from build123d import *

# Parameters (mm, degrees)
SKETCH1_W                = 69.825
SKETCH1_H                = 183.16
FRONT_PLATE_DEPTH        = 1.2
CUT_EXTRUDE1_REACH       = 197.283
SKETCH3_W                = 56.825
SKETCH3_H                = 78.5
SKETCH3_H_2              = 48.66
CONVERT_SOLID5_START     = 1.1684
CONVERT_SOLID5_DEPTH     = 0.0316
M3_CLEARANCE_HOLE1_D     = 3.2
M3_CLEARANCE_HOLE1_DEPTH = 5
M3_CLEARANCE_HOLE1_TIP   = 0.96137699
SKETCH62_W               = 13
SKETCH62_H               = 78.5
BOSS_EXTRUDE2_DEPTH      = 1.1684
FILLET1_R                = 5
M3_CLEARANCE_HOLE2_D     = 3.2
M3_CLEARANCE_HOLE2_DEPTH = 5
M3_CLEARANCE_HOLE2_TIP   = 0.96137699


# Read off the part's stored shape, not the designer's step: Convert-Solid5
with BuildPart() as part:
    # Sketch1 → front_plate (new body)
    with BuildSketch(Plane.XY):
        with Locations((34.9125, -90.788691865)):
            Rectangle(SKETCH1_W, SKETCH1_H)
    extrude(amount=FRONT_PLATE_DEPTH)

    # Sketch3 → Cut-Extrude1 (cut, up to next)
    with BuildSketch(Plane.XY.offset(1.2), mode=Mode.PRIVATE) as cut_extrude1_sk1:
        with Locations((28.4125, -68.458691865)):
            Rectangle(SKETCH3_W, SKETCH3_H)
    cut_extrude1_tool1 = extrude(cut_extrude1_sk1.sketch, amount=-CUT_EXTRUDE1_REACH, mode=Mode.PRIVATE) & part.part
    # Sketch3 → Cut-Extrude1 (cut, up to next)
    with BuildSketch(Plane.XY.offset(1.2), mode=Mode.PRIVATE) as cut_extrude1_sk2:
        with Locations((28.4125, -145.038691865)):
            Rectangle(SKETCH3_W, SKETCH3_H_2)
    cut_extrude1_tool2 = extrude(cut_extrude1_sk2.sketch, amount=-CUT_EXTRUDE1_REACH, mode=Mode.PRIVATE) & part.part
    add(cut_extrude1_tool1.solids().sort_by_distance((28.4125, -68.458692, 1.2))[0], mode=Mode.SUBTRACT)
    add(cut_extrude1_tool2.solids().sort_by_distance((28.4125, -145.038692, 1.2))[0], mode=Mode.SUBTRACT)

    # Convert-Solid5 outline → Convert-Solid5 (cut)
    with BuildSketch(Plane.XY.offset(CONVERT_SOLID5_START)):
        Polygon((56.825, -107.708691865), (0, -107.708691865), (0, -120.708691865), (56.825, -120.708691865), (56.825, -169.368691865), (0, -169.368691865), (0, -182.368691865), (69.825, -182.368691865), (69.825, 0.791308135), (0, 0.791308135), (0, -29.208691865), (56.825, -29.208691865), align=None)
    extrude(amount=CONVERT_SOLID5_DEPTH, mode=Mode.SUBTRACT)

    # M3 Clearance Hole1
    with Locations(Plane.XY.offset(1.1684)):
        with Locations((63.325, -92.708691865), (63.325, -113.708691865), (64.2, -6.233691865), (64.2, -175.343691865)):
            Hole(M3_CLEARANCE_HOLE1_D / 2, depth=M3_CLEARANCE_HOLE1_DEPTH)
            with Locations((0, 0, -(M3_CLEARANCE_HOLE1_DEPTH + M3_CLEARANCE_HOLE1_TIP / 2))):  # 118° drill point
                Cone(0, M3_CLEARANCE_HOLE1_D / 2, M3_CLEARANCE_HOLE1_TIP, mode=Mode.SUBTRACT)

    # Mirror2: part across plane


with BuildPart() as part_1:
    add(part.part)
    add(part.part.mirror(Plane(origin=(0, 0.791308135, 0), x_dir=(0, 0, 1), z_dir=(-1, 0, 0))))

    # Sketch62 → Boss-Extrude2 (add)
    with BuildSketch(Plane.XY.offset(1.1684)):
        with Locations((-8.74, -68.458691865)):
            Rectangle(SKETCH62_W, SKETCH62_H)
    extrude(amount=-BOSS_EXTRUDE2_DEPTH)

    # Fillet1
    fillet1_edges = [part_1.edges().sort_by_distance(p)[0] for p in [
        (-15.24, -107.708691865, 0.5842),
        (-15.24, -29.208691865, 0.5842),
        (-2.24, -29.208691865, 0.5842),
        (-2.24, -107.708691865, 0.5842),
        (56.825, -120.708691865, 0.5842),
        (56.825, -169.368691865, 0.5842),
        (69.825, -182.368691865, 0.5842),
        (69.825, 0.791308135, 0.5842),
        (56.825, -29.208691865, 0.5842),
        (56.825, -107.708691865, 0.5842),
        (-56.825, -107.708691865, 0.5842),
        (-56.825, -29.208691865, 0.5842),
        (-69.825, 0.791308135, 0.5842),
        (-69.825, -182.368691865, 0.5842),
        (-56.825, -169.368691865, 0.5842),
        (-56.825, -120.708691865, 0.5842),
    ]]
    fillet(fillet1_edges, radius=FILLET1_R)

    # M3 Clearance Hole2
    with Locations(Plane.XY.offset(1.1684)):
        with Locations((-8.74, -6.233691865), (-8.74, -59.958691865), (-8.74, -113.708691865)):
            Hole(M3_CLEARANCE_HOLE2_D / 2, depth=M3_CLEARANCE_HOLE2_DEPTH)
            with Locations((0, 0, -(M3_CLEARANCE_HOLE2_DEPTH + M3_CLEARANCE_HOLE2_TIP / 2))):  # 118° drill point
                Cone(0, M3_CLEARANCE_HOLE2_D / 2, M3_CLEARANCE_HOLE2_TIP, mode=Mode.SUBTRACT)


solid = part_1.part
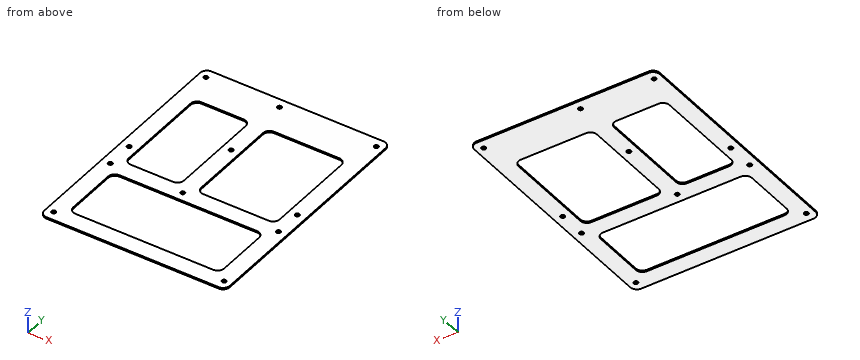
Design review of the part built by this model. Coordinates are the model's own, in mm. Give positions to 0.01 mm unless a question says otherwise; leave off trailing zeros. Loops run counter-clockwise (first coordinate to the right, second up) from the corner with the lowest first, then second, coordinate; pieces in that order, holes last. Notation, with made-up numbers: (12.25, 5.5) - (30.25, 5.5) arc R20 ccw to (30.25, 22.5) - close; hole circle Ø10 at (-5.75, -9.75). An arc over 180 degrees is marked (long way). Use CSV: the item, a comma, the result in double quotes. Start each with the question number.
1. Add section D-D (z = 0.2). Count the separate pieces of the cut face and the enclosed holes in it, plus the area to 3 significant figures.
2. Insertion check: P1, Ø3, axis at x = 63.32, y = -92.71, coming from the -Z side; P2, Ø4, axis at x = -63.32, y = -92.71, coming from the -Z side. Each pin has a flat end and moves straight along its axis. Give the tip position at first contact, or say it passes through.
3. Add section C-C (x = -29.5). State the section outline as (y, z) points, plus the area to 3 significant figures.
4. Wall thickness on L1, parallel to X at y = -65, z = 0.2 (3 decimals); L2, parallel to Y at x = -8.74, z = 0.5; L3, parallel to Y at x = 2.5, z = 0.55: over which ranges is each line inside the solid? List them lowest first.
5. Add section B-B (y = -149). State the section outline as (x, z) points (3 decimals), plus the area to 3 significant figures.
6. Add section A-A (y = -43.5). State the section outline as (x, z) points (3 decimals), plus the area to 3 significant figures.
Results found:
1,separate pieces,"1"
1,enclosed holes,"14"
1,area,"12,100 mm²"
2,P1,"passes through"
2,P2,"stops at z = 0"
3,outline,"(-182.37, 0) - (-169.37, 0) - (-169.37, 1.17) - (-182.37, 1.17) - close; (-120.71, 0) - (-107.71, 0) - (-107.71, 1.17) - (-120.71, 1.17) - close; (-29.21, 0) - (0.79, 0) - (0.79, 1.17) - (-29.21, 1.17) - close"
3,area,"65.4 mm²"
4,L1,"x = -69.825 to -56.825, -15.24 to -2.24, 56.825 to 69.825"
4,L2,"y = -182.37 to -169.37, -120.71 to -115.31, -112.11 to -61.56, -58.36 to -7.83, -4.63 to 0.79"
4,L3,"y = -182.37 to -169.37, -120.71 to -107.7, -29.22 to 0.79"
5,outline,"(-69.825, 0) - (-56.825, 0) - (-56.825, 1.168) - (-69.825, 1.168) - close; (56.825, 0) - (69.825, 0) - (69.825, 1.168) - (56.825, 1.168) - close"
5,area,"30.4 mm²"
6,outline,"(-69.825, 0) - (-56.825, 0) - (-56.825, 1.168) - (-69.825, 1.168) - close; (-15.24, 0) - (-2.24, 0) - (-2.24, 1.168) - (-15.24, 1.168) - close; (56.825, 0) - (69.825, 0) - (69.825, 1.168) - (56.825, 1.168) - close"
6,area,"45.6 mm²"
